Geometry: final body of the model. Coordinates: model frame, mm. A direction names the side the tool comes from. Coordinates: 2 decimals unless noted, no trailing zeros. Write each loop counter-clockwise with the first axis right and the second up, starting at its lowest first coordinate (ties: lowest second). Pieces come first, ordered by that corner, then holes. Notation, with made-up numbers: (1.25, 10) - (30.25, 10) arc R16 cw to (30.25, 19) - close; hole circle Ø4 at (52.25, 27.25). An arc over 180 degrees is marked (long way). Answer as a JSON object with one key per item and string values. Group by question number.
Item 1: Section C-C on y = 5. Return loops of the section in (x, z).
Item 2: Set-up query: faces 1 (the flat face through (0, -3, 0)), 2 (the cylindrical face through (-3.65, 2.8, 9.35)). Return all of +Z, -Z, +X, -X, +Y, -Y with unobstructed straight access to the full face (end or side cutting, diameter ignored); none if empty.
Item 3: Line query: line 1 along Z through (x, y) = (-6, 1); line 2 along Y through (x, z) = (0, 11.25); line 3 along Z through (x, y) = (0, 4.45). Output: solid intervals per line, ascending. Write a range as from..to.
Item 4: First-contact query: pin 1 Ø1 at (y, z) = (-4, 9.5) entering from +X; pin 2 Ø2.5 at (x, z) = (0, 2.9) entering from +Y; pin 3 Ø3 at (x, y) = (0, 0) entering from +Z; pin 4 Ø5 at (y, z) = (5.5, 6.5) entering from +X. Flat tips, straight axial feed; report the tip coordinate or a pass-through.
Item 5: Section A-A on x = 0. Return loops of the section in (y, z), and give its area (3 significant figures).
Item 6: Mould query, pull axis Y, two halves, no side actions, for faces 3 (the cylindrical face through (6.466, 2.681, 2.859)), 4 (the cylindrical face through (-1.5, 4.47, 2.97)), 5 (the cylindrical face through (-0.54, -2.44, 7.1)). Classes: pulls with the +Y half, pulls with the -Y half, needs draft (parallel to the pull), parting line crosses it, or undercut.
Item 7: Section D-D on x = 5.5. Return loops of the section in (y, z), and give its area (3 significant figures).
Item 8: Section B-B on y = 0. Return loops of the section in (x, z).
Solid Edge part; units mm, degrees
sketch "Sketch1" plane through (0, 0, 0) normal (0, 0, 1) x (1, 0, 0)
  circle A0 centre (0, 0) radius 7
extrude "Protrusion1" add sketch "Sketch1" along normal blind 5.8
sketch "Sketch2" plane through (0, 0, 5.8) normal (0, 0, 1) x (1, 0, 0)
  circle A0 centre (0, 0) radius 4.6
extrude "ExtrudedProtrusion_2" add sketch "Sketch2" along normal blind 7.2
sketch "Sketch3" plane through (0, 0, 13) normal (0, 0, 1) x (1, 0, 0)
  circle A0 centre (0, 0) radius 7
extrude "ExtrudedProtrusion_3" add sketch "Sketch3" along normal blind 1
sketch "Sketch4" plane through (0, 0, 0) normal (0, -1, 0) x (1, 0, 0)
  circle A0 centre (0, 2.9) radius 1.5
extrude "ExtrudedCutout_1" cut sketch "Sketch4" against normal blind 115.8762
sketch "Sketch5" plane through (0, 0, 14) normal (0, 0, 1) x (1, 0, 0)
  circle A0 centre (0, 0) radius 2.5
extrude "Cutout1" cut sketch "Sketch5" against normal through all
properties material "ABS Plastic, medium impact"
Checks:
{
 "1": {"outline": "(-4.9, 0) - (4.9, 0) - (4.9, 5.8) - (-4.9, 5.8) - close; (-4.9, 13) - (4.9, 13) - (4.9, 14) - (-4.9, 14) - close; hole circle Ø3 at (0, 2.9)"},
 "2": {"face 1": "-Z, +X, -X, +Y, -Y", "face 2": "none"},
 "3": {"line 1": "0..5.8, 13..14", "line 2": "-4.6..-2.5, 2.5..4.6", "line 3": "0..1.4, 4.4..14"},
 "4": {"pin 1": "x = 2.98", "pin 2": "y = -2.17", "pin 3": "through", "pin 4": "x = 6.28"},
 "5": {"outline": "(-7, 0) - (-2.5, 0) - (-2.5, 14) - (-7, 14) - (-7, 13) - (-4.6, 13) - (-4.6, 5.8) - (-7, 5.8) - close; (2.5, 0) - (7, 0) - (7, 1.4) - (2.5, 1.4) - close; (2.5, 4.4) - (7, 4.4) - (7, 5.8) - (4.6, 5.8) - (4.6, 13) - (7, 13) - (7, 14) - (2.5, 14) - close", "area": "77.9 mm^2"},
 "6": {"face 3": "parting line crosses it", "face 4": "needs draft", "face 5": "undercut"},
 "7": {"outline": "(-4.33, 0) - (4.33, 0) - (4.33, 5.8) - (-4.33, 5.8) - close; (-4.33, 13) - (4.33, 13) - (4.33, 14) - (-4.33, 14) - close", "area": "58.9 mm^2"},
 "8": {"outline": "(-7, 0) - (-2.5, 0) - (-2.5, 14) - (-7, 14) - (-7, 13) - (-4.6, 13) - (-4.6, 5.8) - (-7, 5.8) - close; (2.5, 0) - (7, 0) - (7, 5.8) - (4.6, 5.8) - (4.6, 13) - (7, 13) - (7, 14) - (2.5, 14) - close"}
}
